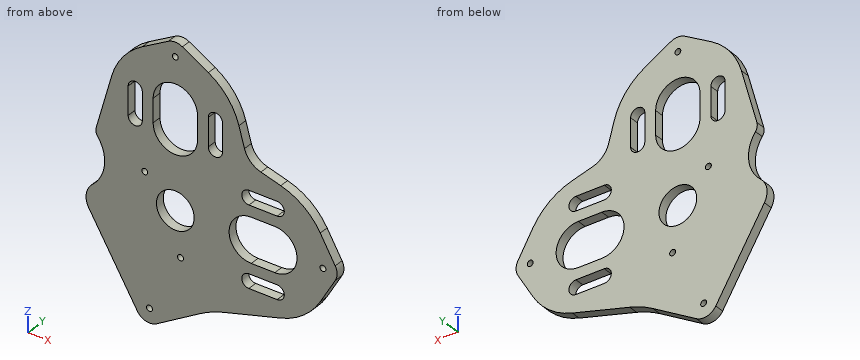
from build123d import *

# Parameters (mm, degrees)
F0_R     = 0.625
F0_R_2   = 4
F1_DEPTH = 2


with BuildPart() as f1:
    # F0 (on Front) → F1 (new body)
    with BuildSketch(Plane.XZ):
        with BuildLine():
            ThreePointArc((-17.552148, -1.263062), (-18.877937, -3.655988), (-18.355769, -6.341347))
            Line((-18.355769, -6.341347), (-8.04557, -23.5004))
            ThreePointArc((-8.04557, -23.5004), (-6.199833, -24.866173), (-3.928953, -24.526788))
            Line((-3.928953, -24.526788), (5.264061, -19.003068))
            ThreePointArc((5.264061, -19.003068), (7.654891, -17.777065), (10.188478, -16.882589))
            Line((10.188478, -16.882589), (22.363441, -13.484677))
            ThreePointArc((22.363441, -13.484677), (27.181397, -11.061629), (30.725984, -6.997178))
            Line((30.725984, -6.997178), (33.898425, -1.499395))
            ThreePointArc((33.898425, -1.499395), (34.3, 0), (33.898425, 1.499395))
            Line((33.898425, 1.499395), (30.725984, 6.997178))
            ThreePointArc((30.725984, 6.997178), (27.181397, 11.061629), (22.363441, 13.484677))
            Line((22.363441, 13.484677), (18.1363, 14.66443))
            ThreePointArc((18.1363, 14.66443), (15.944852, 15.944852), (14.66443, 18.1363))
            Line((14.66443, 18.1363), (13.484677, 22.363441))
            ThreePointArc((13.484677, 22.363441), (11.061629, 27.181397), (6.997178, 30.725984))
            Line((6.997178, 30.725984), (1.499395, 33.898425))
            ThreePointArc((1.499395, 33.898425), (0, 34.3), (-1.499395, 33.898425))
            Line((-1.499395, 33.898425), (-6.997178, 30.725984))
            ThreePointArc((-6.997178, 30.725984), (-11.061629, 27.181397), (-13.484677, 22.363441))
            Line((-13.484677, 22.363441), (-16.76984, 10.592467))
            ThreePointArc((-16.76984, 10.592467), (-16.810073, 9.690932), (-16.449911, 8.863486))
            ThreePointArc((-16.449911, 8.863486), (-15.01815, 3.584383), (-17.552148, -1.263062))
        make_face()
        with Locations((-5.474068, -21.955286)):
            Circle(F0_R, mode=Mode.SUBTRACT)
        with Locations((1.1, -9.184362)):
            Circle(F0_R, mode=Mode.SUBTRACT)
        Circle(F0_R_2, mode=Mode.SUBTRACT)
        with BuildLine():
            Line((18.6, -7), (21.6, -7))
            ThreePointArc((21.6, -7), (23.09998, -8.492292), (21.615416, -9.999921))
            ThreePointArc((21.615416, -9.999921), (21.6, -10), (21.584584, -9.999921))
            Line((21.584584, -9.999921), (18.6, -9.999921))
            Line((18.6, -9.999921), (15.615416, -9.999921))
            Line((15.615416, -9.999921), (15.584584, -9.999921))
            ThreePointArc((15.584584, -9.999921), (14.10002, -8.492292), (15.6, -7))
            Line((15.6, -7), (18.6, -7))
        make_face(mode=Mode.SUBTRACT)
        with BuildLine():
            ThreePointArc((16.1, -4.7), (11.4, 0), (16.1, 4.7))
            Line((16.1, 4.7), (21.1, 4.7))
            ThreePointArc((21.1, 4.7), (25.8, 0), (21.1, -4.7))
            Line((21.1, -4.7), (16.1, -4.7))
        make_face(mode=Mode.SUBTRACT)
        with Locations((31.3, 0)):
            Circle(F0_R, mode=Mode.SUBTRACT)
        with Locations((-6.480741, 5.5)):
            Circle(F0_R, mode=Mode.SUBTRACT)
        with BuildLine():
            ThreePointArc((-9.999921, 21.615416), (-8.492292, 23.09998), (-7, 21.6))
            Line((-7, 21.6), (-7, 18.6))
            Line((-7, 18.6), (-7, 15.6))
            ThreePointArc((-7, 15.6), (-8.492292, 14.10002), (-9.999921, 15.584584))
            ThreePointArc((-9.999921, 15.584584), (-10, 15.6), (-9.999921, 15.615416))
            Line((-9.999921, 15.615416), (-9.999921, 18.6))
            Line((-9.999921, 18.6), (-9.999921, 21.584584))
            ThreePointArc((-9.999921, 21.584584), (-10, 21.6), (-9.999921, 21.615416))
        make_face(mode=Mode.SUBTRACT)
        with BuildLine():
            ThreePointArc((4.7, 16.1), (0, 11.4), (-4.7, 16.1))
            Line((-4.7, 16.1), (-4.7, 21.1))
            ThreePointArc((-4.7, 21.1), (0, 25.8), (4.7, 21.1))
            Line((4.7, 21.1), (4.7, 16.1))
        make_face(mode=Mode.SUBTRACT)
        with Locations((0, 31.3)):
            Circle(F0_R, mode=Mode.SUBTRACT)
        with BuildLine():
            Line((21.584584, 9.999921), (21.615416, 9.999921))
            ThreePointArc((21.615416, 9.999921), (23.09998, 8.492292), (21.6, 7))
            Line((21.6, 7), (18.6, 7))
            Line((18.6, 7), (15.6, 7))
            ThreePointArc((15.6, 7), (14.10002, 8.492292), (15.584584, 9.999921))
            Line((15.584584, 9.999921), (15.615416, 9.999921))
            Line((15.615416, 9.999921), (18.6, 9.999921))
            Line((18.6, 9.999921), (21.584584, 9.999921))
        make_face(mode=Mode.SUBTRACT)
        with BuildLine():
            ThreePointArc((9.999921, 15.584584), (8.492292, 14.10002), (7, 15.6))
            Line((7, 15.6), (7, 18.6))
            Line((7, 18.6), (7, 21.6))
            ThreePointArc((7, 21.6), (8.492292, 23.09998), (9.999921, 21.615416))
            Line((9.999921, 21.615416), (9.999921, 21.584584))
            Line((9.999921, 21.584584), (9.999921, 18.6))
            Line((9.999921, 18.6), (9.999921, 15.615416))
            ThreePointArc((9.999921, 15.615416), (10, 15.6), (9.999921, 15.584584))
        make_face(mode=Mode.SUBTRACT)
    extrude(amount=F1_DEPTH)


solid = f1.part
Build history of the part. All positions in model axes, mm. Give positions to 0.01 mm unless a question says otherwise; leave off trailing zeros. Write each loop counter-clockwise with the first axis right and the second up, starting at its lowest first coordinate (ties: lowest second). Pieces come first, ordered by that corner, then holes. Notation, with made-up numbers: (72, 27.5) - (112, 27.5) arc R23 cw to (112, 63.5) - close; hole circle Ø9 at (55.5, 6). An arc over 180 degrees is marked (long way). Use one line per item in the form item = value. Start each with the question number.
1. Band-saw the part on A-A on z = -3. Write the cut outline in (x, y), plus the area to 3 significant figures.
2. Band-saw the part on D-D on z = 28. Write the cut outline in (x, y).
3. Band-saw the part on C-C on z = -12. Write the cut outline in (x, y), plus the area to 3 significant figures.
4. Band-saw the part on B-B on y = -1.6. Count the separate pieces of the cut face and the enclosed holes in it, plus the area to 3 significant figures.
5. Probe line 1 (Z direction, x = 0, y = -0.6) (3 decimals); line 2 (Z direction, x = 1.1, y = -1.05); line 3 (X direction, y = -1.3, z = 17.5). List the from-to ranges inside material, lowest first. Write a range as [from, to].
6. Drop flat-ended pins along their axis: pin 1 Ø0.6 at (y, z) = (-1, 18.5) entering from +X; pin 2 Ø1 at (y, z) = (-1, 19.5) entering from -X; pin 3 Ø1 at (x, y) = (19.5, -1) entering from -Z; pin 4 Ø6.5 at (x, z) = (0, 0) entering from -Y. Give the stop position or say it passes through.
Conclusion:
q1.outline = (-18.72, -2) - (-2.65, -2) - (-2.65, 0) - (-18.72, 0) - close; (2.65, -2) - (12.48, -2) - (12.48, 0) - (2.65, 0) - close; (24.72, -2) - (33.03, -2) - (33.03, 0) - (24.72, 0) - close
q1.area = 68.4 mm²
q2.outline = (-10.37, -2) - (10.37, -2) - (10.37, 0) - (-10.37, 0) - close
q3.outline = (-14.96, -2) - (25.81, -2) - (25.81, 0) - (-14.96, 0) - close
q3.area = 81.5 mm²
q4.separate_pieces = 1
q4.enclosed_holes = 12
q4.area = 1,550 mm²
q5.line_1 = [-22.166, -4], [4, 11.4], [25.8, 30.675], [31.925, 34.3]
q5.line_2 = [-21.51, -9.81], [-8.56, -3.85], [3.85, 11.53], [25.67, 34.09]
q5.line_3 = [-14.84, -10], [-7, -4.7], [4.7, 7], [10, 14.89]
q6.pin_1 = 14.65
q6.pin_2 = -14.42
q6.pin_3 = -14.42
q6.pin_4 = through
